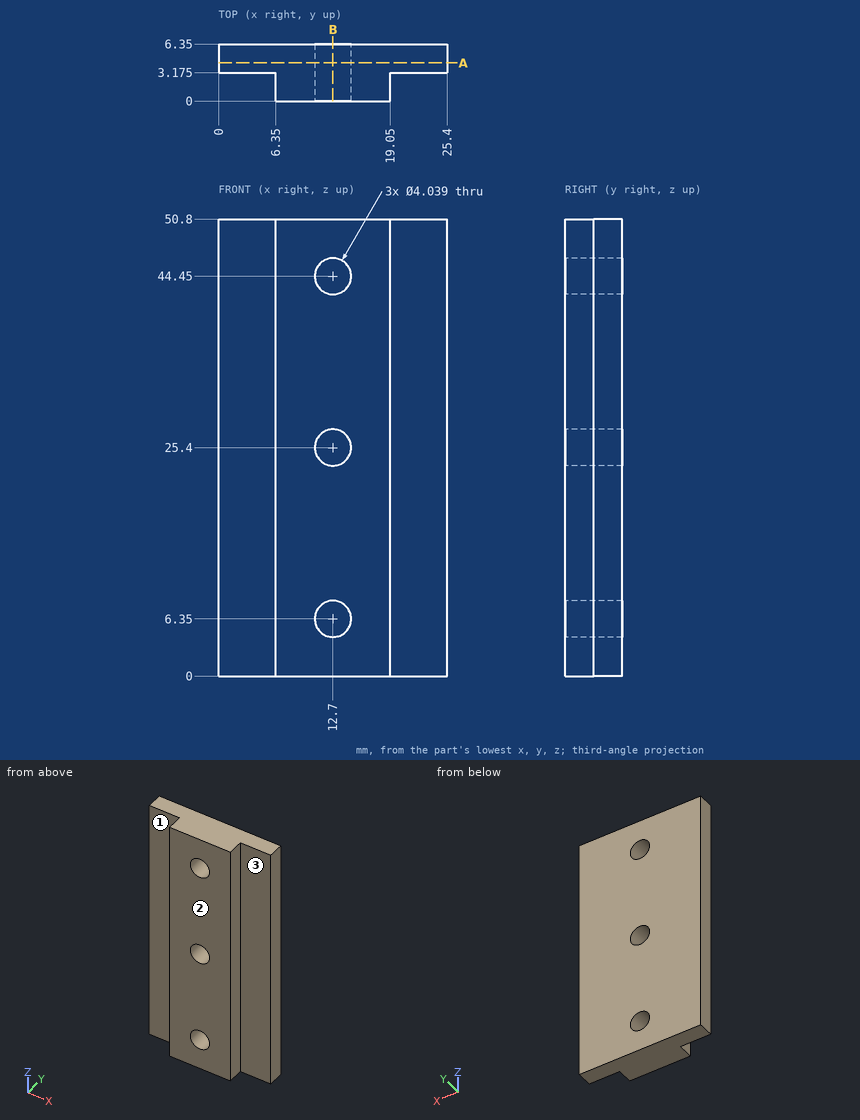
Part print with two shaded views. Sizes in mm from the minimum x, y, z corner. A direction names the side the tool comes from. Round coordinates to 2 decimals unless told otherwise and drop trailing zeros. Write each loop counter-clockwise with the first axis right and the second up, starting at its lowest first coordinate (ties: lowest second). Pieces come first, ordered by that corner, then holes. Notation, with made-up numbers: M 56.5,-5.5 L 73.5,-5.5 A13 cw 73.5,13.5 Z; hole C -12,77.25 d9. An arc over 180 degrees is marked long. Put each result on its own line as item: value. Start each with the question number.
1) Saw through at B-B, the plane x = 12.7. Write the cut outline in (y, z), and give its area (3 significant figures).
2) Pin check, flat tips, straight feed: pin 1 Ø3 at (y, z) = (1.5, 18.5) entering from -X; pin 2 Ø1.9 at (x, z) = (23, 25) entering from -Y (3 decimals). Stop position of each tip, or through.
3) 3-axis set-ups, long thin cutter, end or side, ignore diameter. For the marked faces 1, 2 and 3: which of +Z, -Z, +X, -X, +Y, -Y reach the whole face in a straight line?
4) Saw through at A-A, the plane y = 4.25. Write the cut outline in (x, z), and give its area (3 significant figures).
5) Drill centre lines: probe 1 along Z at (x, y) = (12.7, 2); probe 2 along X at (y, z) = (3.5, 6.5); probe 3 along Z at (x, y) = (12, 4.25) (1 decimal). Where is each one in solid material? Low to high. Write a range as [from, to].
Resolved:
1. outline: M 0,0 L 6.35,0 L 6.35,4.33 L 0,4.33 Z; M 0,8.37 L 6.35,8.37 L 6.35,23.38 L 0,23.38 Z; M 0,27.42 L 6.35,27.42 L 6.35,42.43 L 0,42.43 Z; M 0,46.47 L 6.35,46.47 L 6.35,50.8 L 0,50.8 Z
1. area: 246 mm²
2. pin 1: x = 6.35
2. pin 2: y = 3.175
3. face 1: +Z, -Z, -X, -Y
3. face 2: +Z, -Z, +X, -X, -Y
3. face 3: +Z, -Z, +X, -Y
4. outline: M 0,0 L 25.4,0 L 25.4,50.8 L 0,50.8 Z; hole C 12.7,6.35 d4.04; hole C 12.7,25.4 d4.04; hole C 12.7,44.45 d4.04
4. area: 1,250 mm²
5. probe 1: [0, 4.33], [8.37, 23.38], [27.42, 42.43], [46.47, 50.8]
5. probe 2: [0, 10.69], [14.71, 25.4]
5. probe 3: [0, 4.5], [8.2, 23.5], [27.3, 42.6], [46.3, 50.8]
